Build history of the part. All positions in model axes, mm. A direction names the side the tool comes from. Give positions to 0.01 mm unless a question says otherwise; leave off trailing zeros. Order: outer loops, then holes, each group sorted by start corner. A loop starts at its lowest first (then second) coordinate and runs counter-clockwise, first axis right, second up. Notation, with made-up numbers: (-10.75, -15) - (13.25, -15) arc R16 ccw to (13.25, 8) - close; hole circle Ø8 at (-21, 63). An arc over 180 degrees is marked (long way). Use a Markdown table: item, result. Add a question column.
(1) Slice it at C-C (y = 5.75). Write the cut outline in (x, z), then the cut area to 3 significant figures.
(2) Slice it at D-D (x = 44). Write the cut outline in (y, z).
(3) Flat gauge pins, fed straight in: pin 1 (8 mm diameter, centred on y = 4.5, z = -10.5, fed in from +X); pin 2 (4 mm diameter, centred on x = 71.5, z = -23, fed in from +Y); pin 3 (5 mm diameter, centred on y = 6.5, z = -11, fed in from -X). Where does each tip first touch, or does it go through?
(4) Slice it at B-B (z = -19.5). Write the cut outline in (x, y).
(5) Wall check: line 1 (X direction, y = 1.2, z = -19.5); line 2 (Z direction, x = 71, y = 0.8); line 3 (Y direction, x = 12.5, z = -6.5). Give the ranges that are in metal, low to high.
(6) Mould opens along X. For faces 1 (the face through (-2.92, 1.48, -21.25)), 2 (the face through (34, 9.8, -20)), 3 (the face through (-7.5, 1.5, -19.4)) say: +X half, -X half, draft (parallel to the pull), parting line (faces both ways), or undercut.
(7) Which spindle directions (+Z, -Z, +X, -X, +Y, -Y) get a long thin tool onto all of the face, cutting with end or side? Do faces 4 (the face through (-3.7, 3, -21.3)), 5 (the face through (68, 5, -19)), 6 (the face through (71.8, 3, -21.3)), 7 (the face through (0, 5, -19)). Say none if no direction does.
(8) Slice it at A-A (y = -5.25). Write the cut outline in (x, z).
from build123d import *

# Parameters (mm, degrees)
ESQUISSE1_W        = 68
ESQUISSE1_H        = 39
BOSS_EXTRU_3_DEPTH = 9.8
ESQUISSE5_R        = 1.75
BOSS_EXTRU_5_DEPTH = 3
ESQUISSE6_R        = 1.75
BOSS_EXTRU_6_DEPTH = 3
ESQUISSE7_R        = 0.4
BOSS_EXTRU_7_DEPTH = 8.9
CONG_1_R           = 0.02


with BuildPart() as part:
    # Esquisse1 → Boss.-Extru.3 (new body)
    with BuildSketch(Plane(origin=(0, 0, 0), x_dir=(1, 0, 0), z_dir=(0, 1, 0))):
        with Locations((34, 19.5)):
            Rectangle(ESQUISSE1_W, ESQUISSE1_H)
    extrude(amount=BOSS_EXTRU_3_DEPTH)

    # Esquisse5 → Boss.-Extru.5 (add)
    with BuildSketch(Plane(origin=(0, 0, 0), x_dir=(1, 0, 0), z_dir=(0, 1, 0))):
        with BuildLine():
            Line((0, 27), (0, 12))
            ThreePointArc((0, 12), (-0.878679656, 14.121320344), (-3, 15))
            ThreePointArc((-3, 15), (-7.5, 19.5), (-3, 24))
            ThreePointArc((-3, 24), (-0.878679656, 24.878679656), (0, 27))
        make_face()
        with Locations(Location((-3, 19.5, 0), (0, 0, 270))):
            Circle(ESQUISSE5_R, mode=Mode.SUBTRACT)
    extrude(amount=BOSS_EXTRU_5_DEPTH)

    # Esquisse6 → Boss.-Extru.6 (add)
    with BuildSketch(Plane(origin=(0, 0, 0), x_dir=(1, 0, 0), z_dir=(0, 1, 0))):
        with BuildLine():
            Line((68, 12), (68, 27))
            ThreePointArc((68, 27), (68.878679656, 24.878679656), (71, 24))
            ThreePointArc((71, 24), (75.5, 19.5), (71, 15))
            ThreePointArc((71, 15), (68.878679656, 14.121320344), (68, 12))
        make_face()
        with Locations(Location((71, 19.5, 0), (0, 0, 270))):
            Circle(ESQUISSE6_R, mode=Mode.SUBTRACT)
    extrude(amount=BOSS_EXTRU_6_DEPTH)

    # Esquisse7 → Boss.-Extru.7 (add)
    with BuildSketch(Plane(origin=(0, 0, 0), x_dir=(1, 0, 0), z_dir=(0, 1, 0))):
        with Locations(Location((14, 4, 0), (0, 0, 270))):
            Circle(ESQUISSE7_R)
        with Locations(Location((11.46, 4, 0), (0, 0, 270))):
            Circle(ESQUISSE7_R)
        with Locations(Location((8.92, 4, 0), (0, 0, 270))):
            Circle(ESQUISSE7_R)
        with Locations(Location((6.38, 4, 0), (0, 0, 270))):
            Circle(ESQUISSE7_R)
        with Locations(Location((57, 4, 0), (0, 0, 270))):
            Circle(ESQUISSE7_R)
        with Locations(Location((59.54, 4, 0), (0, 0, 270))):
            Circle(ESQUISSE7_R)
        with Locations(Location((62.08, 4, 0), (0, 0, 270))):
            Circle(ESQUISSE7_R)
    extrude(amount=-BOSS_EXTRU_7_DEPTH)

    # Congé1
    cong_1_edges = [part.edges().sort_by_distance(p)[0] for p in [
        (14, -8.9, -4.4),
        (57, -8.9, -4.4),
        (11.46, -8.9, -4.4),
        (8.92, -8.9, -4.4),
        (6.38, -8.9, -4.4),
        (59.54, -8.9, -4.4),
        (62.08, -8.9, -4.4),
    ]]
    fillet(cong_1_edges, radius=CONG_1_R)


solid = part.part
Solution:
| question | item | result |
|---|---|---|
| 1 | outline | (0, -39) - (68, -39) - (68, 0) - (0, 0) - close |
| 1 | area | 2,650 mm2 |
| 2 | outline | (0, -39) - (9.8, -39) - (9.8, 0) - (0, 0) - close |
| 3 | pin 1 | x = 68.97 |
| 3 | pin 2 | y = 3 |
| 3 | pin 3 | x = 0 |
| 4 | outline | (-7.5, 0) - (-4.75, 0) - (-4.75, 3) - (-7.5, 3) - close; (-1.25, 0) - (69.25, 0) - (69.25, 3) - (68, 3) - (68, 9.8) - (0, 9.8) - (0, 3) - (-1.25, 3) - close; (72.75, 0) - (75.5, 0) - (75.5, 3) - (72.75, 3) - close |
| 5 | line 1 | -7.5 to -4.75, -1.25 to 69.25, 72.75 to 75.5 |
| 5 | line 2 | -24 to -21.25, -17.75 to -15 |
| 5 | line 3 | 0 to 9.8 |
| 6 | face 1 | undercut |
| 6 | face 2 | draft |
| 6 | face 3 | -X half |
| 7 | face 4 | +Z, -Z, -X, +Y |
| 7 | face 5 | +X, +Y |
| 7 | face 6 | +Z, -Z, +X, +Y |
| 7 | face 7 | -X, +Y |
| 8 | outline | circle Ø0.8 at (6.38, -4); circle Ø0.8 at (8.92, -4); circle Ø0.8 at (11.46, -4); circle Ø0.8 at (14, -4); circle Ø0.8 at (57, -4); circle Ø0.8 at (59.54, -4); circle Ø0.8 at (62.08, -4) |
